```python
from build123d import *

# Parameters (mm, degrees)
SKETCH_1_R          = 3
EXTRUDE_1_DEPTH     = 12
FILLET_1_R          = 3
FILLET_2_R          = 3
CUT_EXTRUDE_1_DEPTH = 23
CUT_EXTRUDE_2_DEPTH = 35.467375879
CUT_EXTRUDE_3_DEPTH = 3
CUT_EXTRUDE_START   = -23.50608032
CUT_EXTRUDE_8_DEPTH = 23.50608032


# Read off the part's stored shape, not the designer's step: the extrude step
with BuildPart() as part:
    # Sketch 1 → Extrude 1 (new body)
    with BuildSketch(Plane(origin=(0, 0, 0), x_dir=(1, 0, 0), z_dir=(0, 1, 0))):
        with BuildLine():
            Line((-15, 12), (15, 12))
            Line((15, 12), (15, -12))
            Line((15, -12), (-7, -12))
            ThreePointArc((-7, -12), (-8.996142529, -4.664095019), (-15, 0))
            Line((-15, 0), (-15, 12))
        make_face()
        with Locations(Location((10, -8, 0), (0, 0, 270))):
            Circle(SKETCH_1_R, mode=Mode.SUBTRACT)
        with Locations(Location((-3, -8, 0), (0, 0, 270))):
            Circle(SKETCH_1_R, mode=Mode.SUBTRACT)
    extrude(amount=EXTRUDE_1_DEPTH)

    # Fillet 1
    fillet_1_edges = [part.edges().sort_by_distance(p)[0] for p in [
        (-7, 6, 12),
        (-15, 6, 0),
    ]]
    fillet(fillet_1_edges, radius=FILLET_1_R)

    # Fillet 2
    fillet_2_edges = [part.edges().sort_by_distance(p)[0] for p in [
        (15, 6, 12),
    ]]
    fillet(fillet_2_edges, radius=FILLET_2_R)

    # Sketch 2 → Cut-Extrude 1 (cut)
    with BuildSketch(Plane.ZY.offset(15)):
        Polygon((-12, 6), (-6.32871818, 6), (-6.32871818, 10), (-12, 9), align=None)
        Polygon((-6.32871818, 2), (-6.32871818, 6), (-12, 6), (-12, 3), align=None)
    extrude(amount=-CUT_EXTRUDE_1_DEPTH, mode=Mode.SUBTRACT)

    # Sketch 2_3 → Cut-Extrude 2 (cut, through all)
    with BuildSketch(Plane.ZY.offset(15)):
        with BuildLine():
            Line((-1.956143181, 5.390242862), (-1.956143181, 6))
            Line((-1.956143181, 6), (-5.860925645, 6))
            ThreePointArc((-5.860925645, 6), (-4.169499034, 4.023947758), (-1.956143181, 5.390242862))
        make_face()
        with BuildLine():
            Line((-5.860925645, 6), (-1.956143181, 6))
            Line((-1.956143181, 6), (-1.956143181, 6.609757138))
            ThreePointArc((-1.956143181, 6.609757138), (-4.169499034, 7.976052242), (-5.860925645, 6))
        make_face()
    extrude(amount=-CUT_EXTRUDE_2_DEPTH, mode=Mode.SUBTRACT)

    # Sketch 2_4 → Cut-Extrude 3 (cut)
    with BuildSketch(Plane.ZY.offset(15)):
        with BuildLine():
            ThreePointArc((-1.956143181, 5.390242862), (-4.169499034, 4.023947758), (-5.860925645, 6))
            Line((-5.860925645, 6), (-6.32871818, 6))
            Line((-6.32871818, 6), (-6.32871818, 2))
            ThreePointArc((-6.32871818, 2), (-4.179132798, 1.310784265), (-1.956143181, 1.703279883))
            Line((-1.956143181, 1.703279883), (-1.956143181, 5.390242862))
        make_face()
        with BuildLine():
            Line((-6.32871818, 6), (-5.860925645, 6))
            ThreePointArc((-5.860925645, 6), (-4.169499034, 7.976052242), (-1.956143181, 6.609757138))
            Line((-1.956143181, 6.609757138), (-1.956143181, 10.296720117))
            ThreePointArc((-1.956143181, 10.296720117), (-4.179132798, 10.689215735), (-6.32871818, 10))
            Line((-6.32871818, 10), (-6.32871818, 6))
        make_face()
        with BuildLine():
            ThreePointArc((-1.860925645, 6), (-1.884873402, 5.691426611), (-1.956143181, 5.390242862))
            Line((-1.956143181, 5.390242862), (-1.956143181, 1.703279883))
            ThreePointArc((-1.956143181, 1.703279883), (0.839074355, 6), (-1.956143181, 10.296720117))
            Line((-1.956143181, 10.296720117), (-1.956143181, 6.609757138))
            ThreePointArc((-1.956143181, 6.609757138), (-1.884873402, 6.308573389), (-1.860925645, 6))
        make_face()
    extrude(amount=-CUT_EXTRUDE_3_DEPTH, mode=Mode.SUBTRACT)

    # Cut-Extrude 8 outline → Cut-Extrude 8 (cut)
    with BuildSketch(Plane(origin=(0, 0, -12), x_dir=(-1, 0, 0), z_dir=(0, 0, -1)).offset(CUT_EXTRUDE_START)):
        with BuildLine():
            ThreePointArc((-15.000002785, -5.871e-06), (-13.649110641, 5.99999952), (-15.000002373, 12.000005003))
            Line((-15.000002373, 12.000005003), (-15.000002785, -5.871e-06))
        make_face()
    extrude(amount=CUT_EXTRUDE_8_DEPTH, mode=Mode.SUBTRACT)


solid = part.part
```
Build history of the part. All positions in model axes, mm. A direction names the side the tool comes from. Give positions to 0.01 mm unless a question says otherwise; leave off trailing zeros. Order: outer loops, then holes, each group sorted by start corner. A loop starts at its lowest first (then second) coordinate and runs counter-clockwise, first axis right, second up. Notation, with made-up numbers: M 15.25,-1 L 40.25,-1 A26 cw 40.25,19 Z; hole C 30,46.25 d8. An arc over 180 degrees is marked long. Write item = value, one per line. Start each with the question number.
(1) Pin check, flat tips, straight feed: pin 1 Ø4 at (x, y) = (0.5, 6) entering from -Z; pin 2 Ø9.5 at (x, z) = (10, 8) entering from +Y; pin 3 Ø1.5 at (y, z) = (5, 8.5) entering from +X; pin 4 Ø1.7 at (y, z) = (6, -9) entering from -X. Stop position of each tip, or through.
(2) Slice it at B-B on x = -3. Write the cut outline in (y, z).
(3) Probe L1, parallel to X at y = 3.5, z = 8; L2, parallel to X at y = 5.5, z = 8; L3, parallel to X at y = 6.25, z = -10.25. List the from-to ranges inside material, lowest first. Write a range as [from, to].
(4) Which spindle directions (+Z, -Z, +X, -X, +Y, -Y) get a long thin tool onto all of the face, cutting with end or side? Do faces 1 (the cylindrical face through (-9.176, 5.916, 4.402)), 2 (the flat face through (-2, 6, -6.329)), 3 (the flat face through (-1, 6, -1.956)). Say none if no direction does.
(5) Two-plate mould, pull along Z, no slides. Class faces 4 (the cylindrical face through (8.85, 5.92, 10.77)), 5 (the flat face through (0, 0, -3)), 6 (the cylindrical face through (-14.38, 1.38, -0.13)): released by +Z, released by -Z, zero draft, split by the parting line, or undercut.
(6) Slice it at D-D on y = 2.5. Write the cut outline in (x, z).
(7) Slice it at A-A on x = 10. Write the cut outline in (y, z).
(8) Slice it at C-C on z = 8. Write the cut outline in (x, y).
Responses:
q1.pin_1 = -6.33
q1.pin_2 = 12
q1.pin_3 = 13.76
q1.pin_4 = 8
q2.outline = M 0,-12 L 3,-12 L 2,-6.33 L 10,-6.33 L 9,-12 L 12,-12 L 12,5 L 0,5 Z; M 0,11 L 12,11 L 12,12 L 0,12 Z; hole M 5.39,-1.96 A2 ccw long 6.61,-1.96 Z
q3.L1 = [-7.45, -6], [0, 7], [13, 13.87]
q3.L2 = [-7.45, -6], [0, 7], [13, 13.66]
q3.L3 = [8, 13.65]
q4.face_1 = +Z, -X, +Y, -Y
q4.face_2 = -X
q4.face_3 = +X, -X
q5.face_4 = undercut
q5.face_5 = zero draft
q5.face_6 = released by +Z
q6.outline = M -15,-12 L 14.09,-12 L 14.09,11.15 A3 ccw 12,12 L -4.16,12 A3 ccw -7.13,9.46 A12 cw -13.4,0.7 A3 ccw -14.74,-0.72 L -12,-0.72 L -12,-6.33 L 8,-6.33 L 8,-9.16 L -15,-9.16 Z; hole C -3,8 d6; hole C 10,8 d6
q7.outline = M 0,-12 L 12,-12 L 12,5 L 0,5 Z; M 0,11 L 12,11 L 12,12 L 0,12 Z; hole M 5.39,-1.96 A2 ccw long 6.61,-1.96 Z
q8.outline = M -7.45,0 L -6,0 L -6,12 L -7.45,12 Z; M 0,0 L 7,0 L 7,12 L 0,12 Z; M 13,0 L 15,0 A14 cw 15,12 L 13,12 Z
